```python
from build123d import *

# Parameters (mm, degrees)
P_IDAT_VYSUNUT_M1_DEPTH             = 1
SKICA3_R                            = 0.5
ODEBRAT_VYSUNUT_M1_DEPTH            = 64.02628038
ODEBRAT_VYSUNUT_M2_DEPTH            = 64.02628038
ODEBRAT_VYSUNUT_M2_DEPTH_BACK       = 64.02628038
P_IDAT_VYSUNUT_M2_REACH             = 64.499
P_IDAT_VYSUNUT_M2_DIRECTION_2_REACH = 64.499
ZAOBLIT1_R                          = 5


with BuildPart() as part:
    # Skica2 → Přidat vysunutím1 (new, symmetric)
    with BuildSketch(Plane.XY):
        with BuildLine():
            Line((58.568883798, -5.84497543), (56.281036775, -23.194781077))
            ThreePointArc((56.281036775, -23.194781077), (44.962038089, -21.854387935), (33.611521044, -20.814124588))
            ThreePointArc((33.611521044, -20.814124588), (16.298701423, -17.643643834), (0, -11))
            ThreePointArc((0, -11), (18.591127375, -4.663998517), (38.205152177, -3.63202809))
            ThreePointArc((38.205152177, -3.63202809), (48.399667289, -4.622101799), (58.568883798, -5.84497543))
        make_face()
    extrude(amount=P_IDAT_VYSUNUT_M1_DEPTH, both=True)

    # Skica3 → Odebrat vysunutím1 (cut, through all)
    with BuildSketch(Plane.XY.offset(1)):
        with Locations((41.913528916, -9.991754516)):
            Circle(SKICA3_R)
        with Locations((53.842906505, -11.291735411)):
            Circle(SKICA3_R)
        with BuildLine():
            ThreePointArc((47.737008304, -6.766472197), (46.773837436, -8.500989544), (46.292411943, -10.42569161))
            ThreePointArc((46.292411943, -10.42569161), (46.82013174, -11.090155165), (47.484595295, -10.562435368))
            ThreePointArc((47.484595295, -10.562435368), (47.890006236, -8.941633628), (48.701097493, -7.480987442))
            ThreePointArc((48.701097493, -7.480987442), (48.576310521, -6.641685225), (47.737008304, -6.766472197))
        make_face()
    extrude(amount=-ODEBRAT_VYSUNUT_M1_DEPTH, mode=Mode.SUBTRACT)

    # Skica4 → Odebrat vysunutím2 (cut, two sides: drawn at the far end of the back side and taken through both)
    with BuildSketch(Plane.XY.offset(1).offset(-ODEBRAT_VYSUNUT_M2_DEPTH_BACK)):
        with BuildLine():
            Line((44.91326279, -16.319473776), (44.346696401, -21.790214359))
            ThreePointArc((44.346696401, -21.790214359), (50.318767602, -22.450854723), (56.281036775, -23.194781077))
            Line((56.281036775, -23.194781077), (57.000074411, -17.741985017))
            ThreePointArc((57.000074411, -17.741985017), (50.961632228, -16.988554377), (44.91326279, -16.319473776))
        make_face()
    extrude(amount=ODEBRAT_VYSUNUT_M2_DEPTH + ODEBRAT_VYSUNUT_M2_DEPTH_BACK, mode=Mode.SUBTRACT)

    # Přidat vysunutím2: up to this face of the body (flat: up to its plane)
    p_idat_vysunut_m2_end = Plane(part.part.faces().sort_by_distance((32.156276153, -11.702089795, 1))[0])
    # Skica5 → Přidat vysunutím2 (add, up to the picked face)
    with BuildSketch(Plane.XY, mode=Mode.PRIVATE) as p_idat_vysunut_m2_sk1:
        with BuildLine():
            Line((33.611521044, -20.814124588), (44.295190366, -22.287554412))
            ThreePointArc((44.295190366, -22.287554412), (50.260325363, -22.947427482), (56.215669717, -23.69048981))
            Line((56.215669717, -23.69048981), (56.346403833, -22.699072345))
            ThreePointArc((56.346403833, -22.699072345), (50.37720984, -21.954281964), (44.398202436, -21.292874306))
            Line((44.398202436, -21.292874306), (44.346696401, -21.790214359))
            ThreePointArc((44.346696401, -21.790214359), (38.982163929, -21.268567871), (33.611521044, -20.814124588))
        make_face()
    p_idat_vysunut_m2_tool1 = split(extrude(p_idat_vysunut_m2_sk1.sketch, amount=P_IDAT_VYSUNUT_M2_REACH, mode=Mode.PRIVATE), bisect_by=p_idat_vysunut_m2_end, keep=Keep.BOTH, mode=Mode.PRIVATE)
    add(p_idat_vysunut_m2_tool1.solids().sort_by(Axis((48.409605, -22.295213, 0), (0, 0, 1)))[0])

    # Přidat vysunutím2 direction 2: up to this face of the body (flat: up to its plane)
    p_idat_vysunut_m2_direction_2_end = Plane(part.part.faces().sort_by_distance((32.156276153, -11.702089795, -1))[0])
    # Skica5 → Přidat vysunutím2 direction 2 (add, up to the picked face)
    with BuildSketch(Plane.XY, mode=Mode.PRIVATE) as p_idat_vysunut_m2_direction_2_sk1:
        with BuildLine():
            Line((33.611521044, -20.814124588), (44.295190366, -22.287554412))
            ThreePointArc((44.295190366, -22.287554412), (50.260325363, -22.947427482), (56.215669717, -23.69048981))
            Line((56.215669717, -23.69048981), (56.346403833, -22.699072345))
            ThreePointArc((56.346403833, -22.699072345), (50.37720984, -21.954281964), (44.398202436, -21.292874306))
            Line((44.398202436, -21.292874306), (44.346696401, -21.790214359))
            ThreePointArc((44.346696401, -21.790214359), (38.982163929, -21.268567871), (33.611521044, -20.814124588))
        make_face()
    p_idat_vysunut_m2_direction_2_tool1 = split(extrude(p_idat_vysunut_m2_direction_2_sk1.sketch, amount=-P_IDAT_VYSUNUT_M2_DIRECTION_2_REACH, mode=Mode.PRIVATE), bisect_by=p_idat_vysunut_m2_direction_2_end, keep=Keep.BOTH, mode=Mode.PRIVATE)
    add(p_idat_vysunut_m2_direction_2_tool1.solids().sort_by(Axis((48.409605, -22.295213, 0), (0, 0, -1)))[0])

    # Zaoblit1
    zaoblit1_edges = [part.edges().sort_by_distance(p)[0] for p in [
        (58.568883798, -5.84497543, 0),
    ]]
    fillet(zaoblit1_edges, radius=ZAOBLIT1_R)


solid = part.part
```
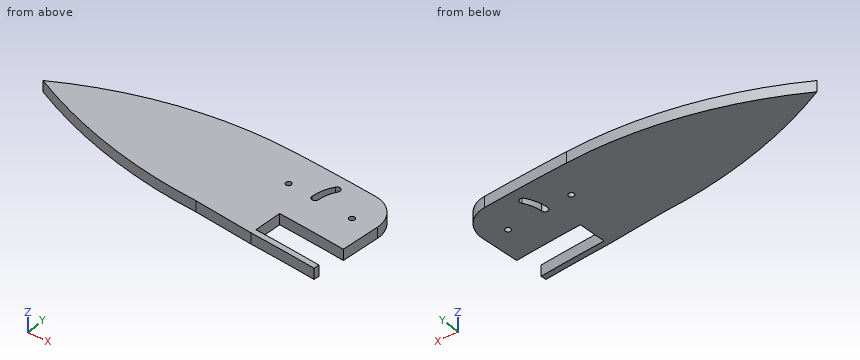
Part model, mm, in its own coordinate system. Round coordinates to 2 decimals unless told otherwise and drop trailing zeros. Loops run counter-clockwise (first coordinate to the right, second up) from the corner with the lowest first, then second, coordinate; pieces in that order, holes last. Notation, with made-up numbers: (84.25, 16.5) -> (137.25, 16.5) arc R17 cw to (137.25, 47.5) -> close; hole circle Ø8 at (5.25, -32.5). An arc over 180 degrees is marked (long way). Use CSV: the item, a comma, the result in double quotes. Start each with the question number.
1) Wall check: L1, parallel to Y at x = 53.5, z = -0.5; L2, parallel to X at y = -9.75, z = 0.6; L3, parallel to Y at x = 25, z = -0.9. Give the ranges that are in metal, low to high. Write a range as [from, to].
2) Cut at B-B, the plane x = 30.5. Write the cut outline in (y, z).
3) Cut at A-A, the plane z = 0.35. Write the cut outline in (x, y), plus the area to 3 significant figures.
4) Cut at C-C, the plane y = -13.75. Write the cut outline in (x, z), plus the area to 3 significant figures.
Determined:
1,L1,"y = [-23.34, -22.33], [-17.29, -11.66], [-10.93, -5.21]"
1,L2,"x = [2.61, 41.48], [42.35, 46.4], [47.63, 57.94]"
1,L3,"y = [-19.7, -3.73]"
2,outline,"(-20.51, -1) -> (-3.39, -1) -> (-3.39, 1) -> (-20.51, 1) -> close"
3,outline,"(0, -11) arc R85.62 ccw to (33.61, -20.81) -> (44.3, -22.29) arc R430 cw to (56.22, -23.69) -> (56.35, -22.7) arc R431 ccw to (44.4, -21.29) -> (44.91, -16.32) arc R436 cw to (57, -17.74) -> (57.91, -10.83) arc R5 ccw to (53.55, -5.21) arc R448 ccw to (38.21, -3.63) arc R71.42 ccw to start; hole circle Ø1 at (41.91, -9.99); hole (46.29, -10.43) arc R0.6 ccw to (47.48, -10.56) arc R6.4 cw to (48.7, -7.48) arc R0.6 ccw to (47.74, -6.77) arc R7.6 ccw to start; hole circle Ø1 at (53.84, -11.29)"
3,area,"739 mm2"
4,outline,"(5.64, -1) -> (57.53, -1) -> (57.53, 1) -> (5.64, 1) -> close"
4,area,"104 mm2"
